Here's how the part is built. I have some questions about the finished solid (model axes, mm). Face numbers are marked on the shaded views. Give positions to 0.01 mm unless a question says otherwise; leave off trailing zeros. Loops run counter-clockwise (first coordinate to the right, second up) from the corner with the lowest first, then second, coordinate; pieces in that order, holes last. Notation, with made-up numbers: M 56.25,83.25 L 78.25,83.25 A26 cw 78.25,109.25 Z; hole C 10.5,55 d2. An arc over 180 degrees is marked long. Answer as CSV lines item,"result". Start each with the question number.
Item 1: I want a section at A-A on y = 97.6. List the corners of the cut face in (x, z) for me.
Item 2: Will these pins go through, and if not, where does the flat tip stop? P1, Ø6, axis at y = 87, z = -15.5, coming from the -X side; P2, Ø1.1, axis at y = -12, z = 3, coming from the -X side; P3, Ø10, axis at y = 95.5, z = -24, coming from the -X side; P4, Ø0.6, axis at y = 42, z = 2.5, coming from the -X side.
Item 3: If we mould it in two halves opening along Z, with no side actions, what happens to the marked faces 1, 2 and 3? For each: released by +Z, released by -Z, zero draft, split by the parting line, or undercut.
Item 4: I want a section at D-D on y = 52. List the corners of the cut face in (x, z) for me, plus the area to 3 significant figures.
Item 5: I want a section at C-C on z = -4.5. List the corners of the cut face in (x, y) for me.
Item 6: I want a section at B-B on y = 1. List the corners of the cut face in (x, z) for me.
Item 7: If I drill on line 1 along Z through (x, y) = (-1, 1); line 2 along X through (y, z) = (97.6, -49.65); line 3 along X through (y, z) = (39, -46), over which ranges is the centre line in solid material (lowest first)? Write a range as from..to.
from build123d import *

# Parameters (mm, degrees)
SKETCH_1_W      = 140
SKETCH_1_H      = 93
PAD_DEPTH       = 5
SKETCH_W        = 140
SKETCH_H        = 7.4
PAD001_DEPTH    = 5
PAD005_DEPTH    = 5
SKETCH002_W     = 9.2
SKETCH002_H     = 9.2
POCKET_DEPTH    = 5
SKETCH004_W     = 2
SKETCH004_H     = 101.4
PAD004_DEPTH    = 51
SKETCH010_W     = 87.7
SKETCH010_H     = 2.08
POCKET003_DEPTH = 11
SKETCH012_W     = 135.8
SKETCH012_H     = 2
PAD006_DEPTH    = 51
PAD007_DEPTH    = 53
SKETCH014_W     = 9.2
SKETCH014_H     = 5
PAD008_DEPTH    = 9.2
SKETCH015_R     = 1.6
POCKET004_DEPTH = 5
SKETCH016_W     = 121.6
SKETCH016_H     = 1.4
PAD009_DEPTH    = 10
CHAMFER_SIZE    = 2
CHAMFER001_SIZE = 0.99
SKETCH017_R     = 3.6
PAD010_DEPTH    = 10
PAD011_DEPTH    = 5
FILLET_R        = 3
SKETCH019_R     = 2
POCKET005_DEPTH = 6.7
PAD012_DEPTH    = 51


with BuildPart() as part:
    # Sketch_1 → Pad (new body)
    with BuildSketch(Plane.XY):
        with Locations((-70, 46.5)):
            Rectangle(SKETCH_1_W, SKETCH_1_H)
    extrude(amount=PAD_DEPTH)

    # Sketch → Pad001 (join)
    with BuildSketch(Plane.XY):
        with Locations((-70, -3.7)):
            Rectangle(SKETCH_W, SKETCH_H)
    extrude(amount=PAD001_DEPTH)

    # Sketch011 (on Face5 of Pad001) → Pad005 (join)
    with BuildSketch(Plane.XY.offset(5)):
        Polygon((-140, 93), (-140, 103.2), (5, 103.2), (5, -7.4), (0, -7.4), (0, 93), align=None)
    extrude(amount=-PAD005_DEPTH)

    # Sketch002 → Pocket (cut)
    with BuildSketch(Plane.XY.offset(5)):
        with Locations((0.4, 98.6)):
            Rectangle(SKETCH002_W, SKETCH002_H)
    extrude(amount=-POCKET_DEPTH, mode=Mode.SUBTRACT)

    # Sketch004 → Pad004 (join)
    with BuildSketch(Plane(origin=(0, 0, 0), x_dir=(1, 0, 0), z_dir=(0, 0, -1))):
        with Locations((4, -43.3)):
            Rectangle(SKETCH004_W, SKETCH004_H)
    extrude(amount=PAD004_DEPTH)

    # Sketch010 → Pocket003 (cut)
    with BuildSketch(Plane(origin=(-140, 0, 0), x_dir=(0, -1, 0), z_dir=(-1, 0, 0))):
        with Locations((-57.4, 2.54)):
            Rectangle(SKETCH010_W, SKETCH010_H)
    extrude(amount=-POCKET003_DEPTH, mode=Mode.SUBTRACT)

    # Sketch012 (on Face10 of Pocket003) → Pad006 (join)
    with BuildSketch(Plane(origin=(0, 0, 0), x_dir=(1, 0, 0), z_dir=(0, 0, -1))):
        with Locations((-72.1, -102.2)):
            Rectangle(SKETCH012_W, SKETCH012_H)
    extrude(amount=PAD006_DEPTH)

    # Sketch013 (on Face10 of Pad006) → Pad007 (join)
    with BuildSketch(Plane(origin=(0, 0, 0), x_dir=(1, 0, 0), z_dir=(0, 0, -1))):
        Polygon((-4.2, -101.2), (-6.2, -101.2), (-6.2, -92), (3, -92), (3, -94), (-4.2, -94), align=None)
    extrude(amount=PAD007_DEPTH)

    # Sketch014 (on Face33 of Pad007) → Pad008 (join)
    with BuildSketch(Plane(origin=(0, 94, 0), x_dir=(-1, 0, 0), z_dir=(0, 1, 0))):
        with Locations((-0.4, -48.5)):
            Rectangle(SKETCH014_W, SKETCH014_H)
    extrude(amount=PAD008_DEPTH)

    # Sketch015 (on Face43 of Pad008) → Pocket004 (cut)
    with BuildSketch(Plane.XY.offset(-46)):
        with Locations((-0.6, 97.6)):
            Circle(SKETCH015_R)
    extrude(amount=-POCKET004_DEPTH, mode=Mode.SUBTRACT)

    # Sketch016 (on Face20 of Pocket004) → Pad009 (join)
    with BuildSketch(Plane.XZ.offset(7.4)):
        with Locations((-58, 2.64)):
            Rectangle(SKETCH016_W, SKETCH016_H)
    extrude(amount=PAD009_DEPTH)

    # Chamfer
    chamfer_edges = [part.edges().sort_by_distance(p)[0] for p in [
        (5, 43.3, 5),
        (-72.1, 103.2, 5),
    ]]
    chamfer(chamfer_edges, length=CHAMFER_SIZE)

    # Chamfer001
    chamfer001_edges = [part.edges().sort_by_distance(p)[0] for p in [
        (-4.2, 97.6, 5),
        (-0.6, 94, 5),
    ]]
    chamfer(chamfer001_edges, length=CHAMFER001_SIZE)

    # Sketch017 (on Face42 of Chamfer001) → Pad010 (join)
    with BuildSketch(Plane(origin=(3, 0, 0), x_dir=(0, -1, 0), z_dir=(-1, 0, 0))):
        with Locations((-88, -17)):
            Circle(SKETCH017_R)
        with Locations((-1, -17)):
            Circle(SKETCH017_R)
    extrude(amount=PAD010_DEPTH)

    # Sketch018 (on Face42 of Pad010) → Pad011 (join)
    with BuildSketch(Plane(origin=(3, 0, 0), x_dir=(0, -1, 0), z_dir=(-1, 0, 0))):
        with BuildLine():
            Line((-85.006674, -15), (-3.993326, -15))
            ThreePointArc((-3.993326, -15), (-4.6, -17), (-3.993326, -19))
            Line((-85.006674, -19), (-3.993326, -19))
            ThreePointArc((-85.006674, -19), (-84.4, -17), (-85.006674, -15))
        make_face()
    extrude(amount=PAD011_DEPTH)

    # Fillet
    fillet_edges = [part.edges().sort_by_distance(p)[0] for p in [
        (3, 44.5, -19),
        (3, 91.6, -17),
        (3, -0.044994, -20.444994),
        (3, 44.5, -15),
        (3, -0.044994, -13.555006),
    ]]
    fillet(fillet_edges, radius=FILLET_R)

    # Sketch019 (on Face32 of Fillet) → Pocket005 (cut)
    with BuildSketch(Plane(origin=(-7, 0, 0), x_dir=(0, -1, 0), z_dir=(-1, 0, 0))):
        with Locations((-88, -17)):
            Circle(SKETCH019_R)
        with Locations((-1, -17)):
            Circle(SKETCH019_R)
    extrude(amount=-POCKET005_DEPTH, mode=Mode.SUBTRACT)

    # Sketch020 (on Face26 of Pocket005) → Pad012 (join)
    with BuildSketch(Plane(origin=(0, 0, 0), x_dir=(1, 0, 0), z_dir=(0, 0, -1))):
        Polygon((-140, -101.2), (-142, -101.2), (-142, -100.2), (-138.5, -100.2), (-137.5, -101.2), (-138.5, -101.2), align=None)
    extrude(amount=PAD012_DEPTH)


solid = part.part
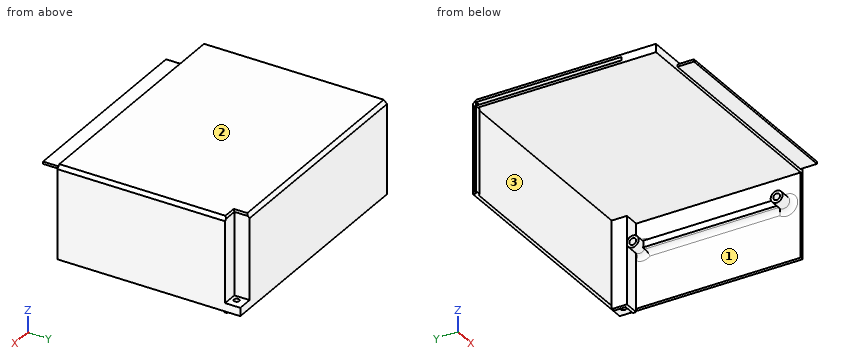
Result:
1,outline,"M -140,0 L -6.2,0 L -6.2,-53 L -4.2,-53 L -4.2,-51 L -2.2,-51 L -2.2,-46 L -4.2,-46 L -4.2,4.01 L -5.19,5 L -140,5 L -140,3.58 L -129,3.58 L -129,1.5 L -140,1.5 Z; M 1,-51 L 5,-51 L 5,-46 L 1,-46 Z"
2,P1,"x = -7"
2,P2,"x = -118.8"
2,P3,"x = -142"
2,P4,"x = -129"
3,face 1,"undercut"
3,face 2,"released by +Z"
3,face 3,"zero draft"
4,outline,"M -140,0 L 3,0 L 3,-12 A3 cw 0,-15 L -2,-15 L -2,-19 L 0,-19 A3 cw 3,-22 L 3,-51 L 5,-51 L 5,3 L 3,5 L -140,5 L -140,3.58 L -129,3.58 L -129,1.5 L -140,1.5 Z"
4,area,"826 mm^2"
5,outline,"M -142,100.2 L -138.5,100.2 L -137.5,101.2 L -6.2,101.2 L -6.2,92 L 3,92 L 3,-7.4 L 5,-7.4 L 5,94 L -4.2,94 L -4.2,103.2 L -140,103.2 L -140,101.2 L -142,101.2 Z"
6,outline,"M -140,0 L 3,0 L 3,-10.4 A3 cw 0,-13.4 L -7,-13.4 L -7,-15 L -0.3,-15 L -0.3,-19 L -7,-19 L -7,-20.6 L 0,-20.6 A3 cw 3,-23.6 L 3,-51 L 5,-51 L 5,3 L 3,5 L -140,5 Z"
7,line 1,"-20.6..-19, -15..-13.4, 0..5"
7,line 2,"-6.2..-2.2, 1..5"
7,line 3,"3..5"
